Geometry: final body of the model. Coordinates: model frame, mm. Give positions to 0.01 mm unless a question says otherwise; leave off trailing zeros. Write each loop counter-clockwise with the first axis right and the second up, starting at its lowest first coordinate (ties: lowest second). Pieces come first, ordered by that corner, then holes. Notation, with made-up numbers: M -32,26.25 L 27,26.25 A16 ccw 27,35.25 Z; hole C -30.75,-16.75 d8. An arc over 180 degrees is marked long. Use a Markdown table: item, result. Add a question column.
(1) Cut plane C-C (x = 1.5). Output: boundary loops of the cut face in (y, z).
(2) Cut plane B-B (y = -1.25). Output: boundary loops of the cut face in (x, z), plus the area to 3 significant figures.
(3) Cut plane A-A (z = 0.15). Output: boundary loops of the cut face in (x, y), plus the area to 3 significant figures.
(4) Material intervals for L1, parallel to Y at x = 2.25, z = 0.1; L2, parallel to X at y = -0.75, z = 0.1; L3, parallel to X at y = -0.35, z = 0, sorted ascending.
Autodesk Inventor part; units mm, degrees
ref_plane "IP_PIN_XY" through (0, 0, 0) normal (1, 0, 0) x (0, 0, -1)
ref_plane "IP_PIN_YZ" through (0, 0, 0) normal (0, 0, -1) x (0, 1, 0)
ref_plane "IP_PIN_ZX" through (0, 0, 0) normal (0, 1, 0) x (1, 0, 0)
sketch "Sketch_2" plane through (0, 0, 0) normal (0, 0, 1) x (1, 0, 0)
  line L0 (-0.5, -0.25) -> (3.8, -0.25)
  line L1 (3.8, -0.25) -> (4, -0.05)
  line L2 (4, -0.05) -> (4, 0.05)
  line L3 (4, 0.05) -> (3.8, 0.25)
  line L4 (3.8, 0.25) -> (-0.5, 0.25)
  line L5 (-0.5, 0.25) -> (-0.5, -0.25)
extrude "Extrusion1" add sketch "Sketch_2" along normal mid plane 0.5
sketch "Sketch_3" plane through (0, 0, 0) normal (0, 0, 1) x (1, 0, 0)
  line L0 (-3.25, -3.6) -> (-3.05, -3.8)
  line L1 (-3.05, -3.8) -> (-2.95, -3.8)
  line L2 (-2.95, -3.8) -> (-2.75, -3.6)
  line L3 (-2.75, -3.6) -> (-2.75, -0.65)
  arc A0 (-2.35, -0.25) -> (-2.75, -0.65) centre (-2.35, -0.65) ccw
  line L4 (-2.35, -0.25) -> (-0.5, -0.25)
  line L5 (-0.5, -0.25) -> (-0.5, 0.25)
  line L6 (-0.5, 0.25) -> (-2.35, 0.25)
  arc A1 (-2.35, 0.25) -> (-3.25, -0.65) centre (-2.35, -0.65) ccw
  line L7 (-3.25, -0.65) -> (-3.25, -3.6)
extrude "Extrusion2" add sketch "Sketch_3" along normal mid plane 0.5
sketch "Sketch_4" plane through (0, 0, 0) normal (0, 1, 0) x (-1, 0, 0)
  line L0 (-3.7, -1.25) -> (-3.7, -0.25)
  line L1 (-3.7, -0.25) -> (-3.8, -0.25)
  line L2 (-3.8, -0.25) -> (-4, -0.05)
  line L3 (-4, -0.05) -> (-4, 0.05)
  line L4 (-4, 0.05) -> (-3.8, 0.25)
  line L5 (-3.8, 0.25) -> (-3.7, 0.25)
  line L6 (-3.7, 0.25) -> (-3.7, 1.25)
  line L7 (-3.7, 1.25) -> (-5, 1.25)
  line L8 (-5, 1.25) -> (-5, -1.25)
  line L9 (-5, -1.25) -> (-3.7, -1.25)
extrude "Extrusion3" cut sketch "Sketch_4" along normal mid plane 0.5
sketch "Sketch_5" plane through (0, 0, 0) normal (1, 0, 0) x (0, 1, 0)
  line L0 (-4, 0.45) -> (-4, -0.45)
  line L1 (-4, -0.45) -> (-3.5, -0.45)
  line L2 (-3.5, -0.45) -> (-3.5, -0.25)
  line L3 (-3.5, -0.25) -> (-3.6, -0.25)
  line L4 (-3.6, -0.25) -> (-3.8, -0.05)
  line L5 (-3.8, -0.05) -> (-3.8, 0.05)
  line L6 (-3.8, 0.05) -> (-3.6, 0.25)
  line L7 (-3.6, 0.25) -> (-3.5, 0.25)
  line L8 (-3.5, 0.25) -> (-3.5, 0.45)
  line L9 (-3.5, 0.45) -> (-4, 0.45)
extrude "Extrusion4" cut sketch "Sketch_5" against normal blind 3.5
ref_plane "IP_PIN_XY" through (0, 0, 0) normal (1, 0, 0) x (0, 0, -1)
ref_plane "IP_PIN_YZ" through (0, 0, 0) normal (0, 0, -1) x (0, 1, 0)
ref_plane "IP_PIN_ZX" through (0, 0, 0) normal (0, 1, 0) x (1, 0, 0)
properties part number "BF021-06-A-B-0400-0280-N-G_P"
Answer list:
| question | item | result |
|---|---|---|
| 1 | outline | M -0.25,-0.25 L 0.25,-0.25 L 0.25,0.25 L -0.25,0.25 Z |
| 2 | outline | M -3.25,-0.25 L -2.75,-0.25 L -2.75,0.25 L -3.25,0.25 Z |
| 2 | area | 0.250 mm² |
| 3 | outline | M -3.25,-3.6 L -3.15,-3.7 L -2.85,-3.7 L -2.75,-3.6 L -2.75,-0.65 A0.4 cw -2.35,-0.25 L 3.8,-0.25 L 3.9,-0.15 L 3.9,0.15 L 3.8,0.25 L -2.35,0.25 A0.9 ccw -3.25,-0.65 Z |
| 3 | area | 5.14 mm² |
| 4 | L1 | -0.25 to 0.25 |
| 4 | L2 | -3.25 to -2.75 |
| 4 | L3 | -3.2 to -2.61 |
